Verification items for the finished model (mm, model axes). Face numbers are marked on the shaded views. A direction names the side the tool comes from. Round coordinates to 2 decimals unless told otherwise and drop trailing zeros. Order: outer loops, then holes, each group sorted by start corner. A loop starts at its lowest first (then second) coordinate and runs counter-clockwise, first axis right, second up. Notation, with made-up numbers: M -8,84.25 L 32,84.25 A25 ccw 32,112.25 Z; hole C -31.75,64 d1. An arc over 180 degrees is marked long. Use one line per item in the form item = value. Start each with the question number.
Item 1: Cross-section at D-D on y = -24.5. Enter the section's corners in (x, z).
Item 2: Tool access check on the marked faces 1 and 2. Record the directions out of +Z, -Z, +X, -X, +Y, -Y that give a thin tool (end or side, any length) a straight path to the whole face; none if there is none.
Item 3: Go/stop test with flat-tipped pins: pin 1 Ø2 at (x, z) = (-13.5, 38) entering from +Y; pin 2 Ø6 at (y, z) = (-12, 15.5) entering from +X. Record where each tip stops, or that it passes through.
Item 4: Cross-section at A-A on y = -5.5. Enter the section's corners in (x, z).
Item 5: Release check for a two-part mould opening along Z. For the marked faces 3, 4 and 5 record: +Z half, -Z half, draft (parallel to the pull), parting line (faces both ways), or undercut.
Item 6: Cross-section at B-B on z = 25.45. Enter the section's corners in (x, y), then the cut area to 3 significant figures.
Item 7: Cross-section at C-C on x = -9. Enter the section's corners in (y, z).
Item 8: Thickness scan on probe 1 along Z at (x, y) = (5.5, -7); probe 2 along X at (y, z) = (-31.5, 25.45); probe 3 along Y at (x, z) = (-3.5, 10). Record the ranges inside material, lowest first. Write a range as [from, to].
from build123d import *

# Parameters (mm, degrees)
SKETCH3_R               = 3.175
BOSS_EXTRUDE2_DEPTH     = 50.9
SKETCH7_W               = 38.4
SKETCH7_H               = 44.4
CUT_EXTRUDE1_DEPTH      = 26.45
F_1_4_20_TAPPED_HOLE1_D = 5.1054


with BuildPart() as part:
    # Sketch3 → Boss-Extrude2 (new body)
    with BuildSketch(Plane.XY):
        with BuildLine():
            Line((-17.009907165, -36.719884412), (8.440092835, -36.719884412))
            Line((8.440092835, -36.719884412), (8.440092835, 14.005115588))
            ThreePointArc((8.440092835, 14.005115588), (-4.284907165, 26.730115588), (-17.009907165, 14.005115588))
            Line((-17.009907165, 14.005115588), (-17.009907165, -36.719884412))
        make_face()
        with Locations((-4.284907165, 14.005115588)):
            Circle(SKETCH3_R, mode=Mode.SUBTRACT)
    extrude(amount=BOSS_EXTRUDE2_DEPTH)

    # Sketch7 → Cut-Extrude1 (cut, through all)
    with BuildSketch(Plane(origin=(8.440092835, 0, 0), x_dir=(0, 0, -1), z_dir=(1, 0, 0))):
        with Locations((-25.45, 4.530115588)):
            Rectangle(SKETCH7_W, SKETCH7_H)
    extrude(amount=-CUT_EXTRUDE1_DEPTH, mode=Mode.SUBTRACT)

    # 1/4-20 Tapped Hole1 (through all)
    with Locations(Plane(origin=(-4.284907165, -36.719884412, 25.45), x_dir=(0, 0, -1), z_dir=(0, -1, 0))):
        with Locations((0, 0)):
            Hole(F_1_4_20_TAPPED_HOLE1_D / 2)


solid = part.part
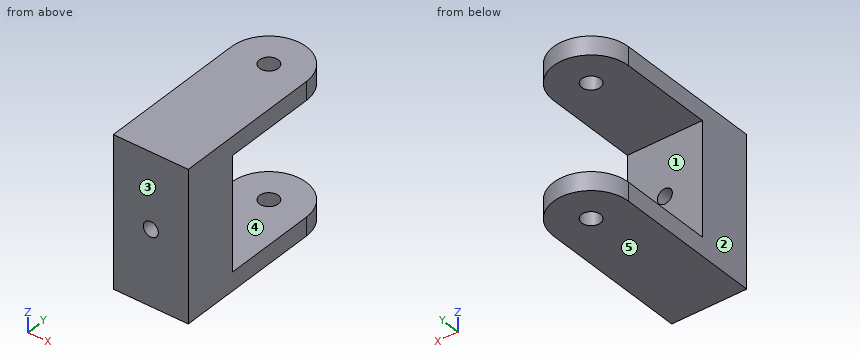
Output values:
q1.outline = M -17.01,0 L 8.44,0 L 8.44,50.9 L -17.01,50.9 Z; hole C -4.28,25.45 d5.11
q2.face_1 = +X, -X, +Y
q2.face_2 = +Z, -Z, -X, +Y, -Y
q3.pin_1 = -17.67
q3.pin_2 = through
q4.outline = M -17.01,0 L 8.44,0 L 8.44,6.25 L -17.01,6.25 Z; M -17.01,44.65 L 8.44,44.65 L 8.44,50.9 L -17.01,50.9 Z
q5.face_3 = draft
q5.face_4 = undercut
q5.face_5 = -Z half
q6.outline = M -17.01,-36.72 L -6.84,-36.72 L -6.84,-17.67 L -17.01,-17.67 Z; M -1.73,-36.72 L 8.44,-36.72 L 8.44,-17.67 L -1.73,-17.67 Z
q6.area = 388 mm2
q7.outline = M -36.72,0 L 25.82,0 L 25.82,6.25 L -17.67,6.25 L -17.67,44.65 L 25.82,44.65 L 25.82,50.9 L -36.72,50.9 Z
q8.probe_1 = [0, 6.25], [44.65, 50.9]
q8.probe_2 = [-17.01, -6.84], [-1.73, 8.44]
q8.probe_3 = [-36.72, -17.67]
